The listing builds one solid part. Answer for the finished solid, in the listing's coordinates (mm). Face numbers are marked on the shaded views. A direction names the side the tool comes from. Coordinates: 2 decimals unless noted, no trailing zeros. Write each loop counter-clockwise with the first axis right and the second up, starting at its lowest first coordinate (ties: lowest second). Pieces come first, ordered by that corner, then holes. Notation, with made-up numbers: M 75.25,-32.5 L 87.25,-32.5 A10 cw 87.25,-21.5 Z; hole C 27,60.5 d3. An arc over 180 degrees is marked long. Put each result on its own line as item: value. Start each with the question number.
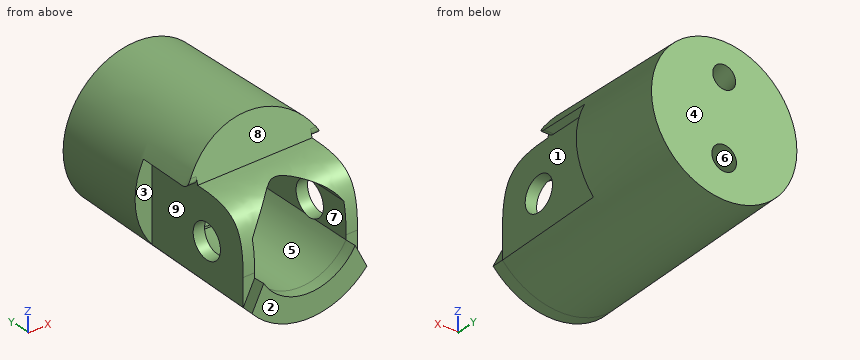
```python
from build123d import *
from build123d.topology import SkipClean

# Parameters (mm, degrees)
SKETCH1_R                     = 6.5
BOSS_EXTRUDE1_DEPTH           = 18
BOSS_EXTRUDE1_TAPER           = 1
BOSS_EXTRUDE1_OTHER_WAY_DEPTH = 10
BOSS_EXTRUDE1_OTHER_WAY_TAPER = -1
SKETCH2_W                     = 5.545055897
SKETCH2_H                     = 10
CUT_EXTRUDE1_DEPTH            = 22.497594206
CUT_EXTRUDE2_DEPTH            = 23.378552983
CUT_EXTRUDE2_DEPTH_BACK       = 23.378552983
CUT_EXTRUDE3_DEPTH            = 23.378552983
CUT_EXTRUDE3_DEPTH_BACK       = 23.378552983
SKETCH4_R                     = 1.5
FILLET1_SIZE                  = 5
CUT_EXTRUDE4_DEPTH            = 21.268192633
CUT_EXTRUDE4_DEPTH_BACK       = 21.268192633
SKETCH5_W                     = 18.469746175
SKETCH5_H                     = 12.695602453
CUT_EXTRUDE5_DEPTH            = 10
BOSS_EXTRUDE3_DEPTH           = 1
BOSS_EXTRUDE3_DRAFT           = -1
SKETCH11_R                    = 1.5
CUT_EXTRUDE7_DEPTH            = 15.423347107
CUT_EXTRUDE7_DRAFT            = -3
SKETCH12_R                    = 1.5
SKETCH13_R                    = 1


with BuildPart() as part:
    # Sketch1 → Boss-Extrude1 (new body)
    with BuildSketch(Plane(origin=(0, 0, 0), x_dir=(1, 0, 0), z_dir=(0, 1, 0))):
        Circle(SKETCH1_R)
    extrude(amount=BOSS_EXTRUDE1_DEPTH, taper=BOSS_EXTRUDE1_TAPER)

    # Sketch1 → Boss-Extrude1 other way (add)
    with BuildSketch(Plane(origin=(0, 0, 0), x_dir=(1, 0, 0), z_dir=(0, 1, 0))):
        Circle(SKETCH1_R)
    extrude(amount=-BOSS_EXTRUDE1_OTHER_WAY_DEPTH, taper=BOSS_EXTRUDE1_OTHER_WAY_TAPER)

    # Sketch2 → Cut-Extrude1 (cut, through all)
    with BuildSketch(Plane.XY.offset(3)):
        with Locations((-7.772527949, -5)):
            Rectangle(SKETCH2_W, SKETCH2_H)
        with Locations((7.772527949, -5)):
            Rectangle(SKETCH2_W, SKETCH2_H)
    extrude(amount=-CUT_EXTRUDE1_DEPTH, mode=Mode.SUBTRACT)

    # Sketch3 → Cut-Extrude2 (cut, two sides: drawn at the far end of the back side and taken through both)
    with BuildSketch(Plane(origin=(5, 0, 0), x_dir=(0, 0, -1), z_dir=(1, 0, 0)).offset(-CUT_EXTRUDE2_DEPTH_BACK)):
        Polygon((-3, -10), (-3, -5), (-18.921941618, -0.733728602), (-18.921941618, -10), align=None)
    extrude(amount=CUT_EXTRUDE2_DEPTH + CUT_EXTRUDE2_DEPTH_BACK, mode=Mode.SUBTRACT)

    # Sketch4 → Cut-Extrude3 (cut, two sides: drawn at the far end of the back side and taken through both)
    with BuildSketch(Plane(origin=(5, 0, 0), x_dir=(0, 0, -1), z_dir=(1, 0, 0)).offset(-CUT_EXTRUDE3_DEPTH_BACK)):
        with Locations(Location((1, -6, 0), (0, 0, 270))):
            Circle(SKETCH4_R)
    extrude(amount=CUT_EXTRUDE3_DEPTH + CUT_EXTRUDE3_DEPTH_BACK, mode=Mode.SUBTRACT)

    # Fillet1
    # a fillet whose section is not a circle: 5 mm, written as the material it takes off along each edge
    with BuildSketch(Plane(origin=(17.5, -10, 3), x_dir=(0, 0, -1), z_dir=(-1, 0, 0))) as fillet1_piece_1:
        with BuildLine():
            Bezier((FILLET1_SIZE, 0), (0, 0), (0, -FILLET1_SIZE), weights=[1, 1.5, 1])
            Line((0, -FILLET1_SIZE), (0, 0))
            Line((0, 0), (FILLET1_SIZE, 0))
        make_face()
    extrude(amount=35, mode=Mode.SUBTRACT)

    # Fillet2
    # a fillet whose section is not a circle: 10, 5 mm, written as the material it takes off along each edge
    with BuildSketch(Plane(origin=(0, 18, 0), x_dir=(1, 0, 0), z_dir=(0, 0, -1))) as fillet2_piece_1:
        with BuildLine():
            Bezier((6.358836316, 9.912737968), (6.185808831, 0), (1.35959784, 0), weights=[1, 0.818181818, 1])
            Line((1.35959784, 0), (6.185808831, 0))
            Line((6.185808831, 0), (6.358836316, 9.912737968))
        make_face()
    revolve(axis=Axis((0, 18, 0), (0, -1, 0)), mode=Mode.SUBTRACT)

    # Sketch5 → Cut-Extrude4 (cut, two sides: drawn at the far end of the back side and taken through both)
    with BuildSketch(Plane(origin=(0, 0, 0), x_dir=(0, 0, -1), z_dir=(1, 0, 0)).offset(-CUT_EXTRUDE4_DEPTH_BACK)):
        with Locations((0.914582981, 14.435063259)):
            Rectangle(SKETCH5_W, SKETCH5_H)
    extrude(amount=CUT_EXTRUDE4_DEPTH + CUT_EXTRUDE4_DEPTH_BACK, mode=Mode.SUBTRACT)

    # Sketch6 → Cut-Extrude5 (cut)
    with BuildSketch(Plane.XZ.offset(10)):
        with BuildLine():
            Line((-4, -2.418971635), (-4, 0.581028365))
            ThreePointArc((-4, 0.581028365), (0, 2.836607379), (4, 0.581028365))
            Line((4, 0.581028365), (4, -2.418971635))
            ThreePointArc((4, -2.418971635), (0, -4.674550649), (-4, -2.418971635))
        make_face()
    extrude(amount=-CUT_EXTRUDE5_DEPTH, mode=Mode.SUBTRACT)

    # Fillet3
    # a fillet whose section is not a circle: 0.5 mm, written as the material it takes off along each edge
    with BuildSketch(Plane(origin=(5, -5, 3), x_dir=(0, 1, 0), z_dir=(1, 0, 0))) as fillet3_piece_1:
        with BuildLine():
            Bezier((0.651612686, 0), (0, 0), (0.168649773, 0.629409523), weights=[1, 1, 1])
            Line((0.168649773, 0.629409523), (0, 0))
            Line((0, 0), (0.651612686, 0))
        make_face()
    extrude(amount=2.493517729, mode=Mode.SUBTRACT)
    with BuildSketch(Plane(origin=(-7.493517729, -5, 3), x_dir=(0, 0.258819045102518, 0.9659258262890691), z_dir=(1, 0, 0))) as fillet3_piece_2:
        with BuildLine():
            Bezier((0.651612686, 0), (0, 0), (0.168649773, -0.629409523), weights=[1, 1, 1])
            Line((0.168649773, -0.629409523), (0, 0))
            Line((0, 0), (0.651612686, 0))
        make_face()
    extrude(amount=2.493517729, mode=Mode.SUBTRACT)


with BuildPart() as boss_extrude3_tool:
    # Sketch9 → Boss-Extrude3 (with draft: the straight prism first)
    with BuildSketch(Plane.XZ.offset(10)):
        with BuildLine():
            Line((-4, -2.418971635), (-5, -4.421495943))
            ThreePointArc((-5, -4.421495943), (0, -6.674550649), (5, -4.421495943))
            Line((5, -4.421495943), (4, -2.418971635))
            ThreePointArc((4, -2.418971635), (0, -4.674550649), (-4, -2.418971635))
        make_face()
    extrude(amount=BOSS_EXTRUDE3_DEPTH)
    # Boss-Extrude3: the draft: its side faces are tilted about the plane it starts from
    boss_extrude3_sides = [boss_extrude3_tool.faces().sort_by_distance(p)[0] for p in [
        (0, -10.5, -6.674550649),
        (4.5, -10.5, -3.420233789),
        (0, -10.5, -4.674550649),
        (-4.5, -10.5, -3.420233789),
    ]]
    draft(boss_extrude3_sides, Plane.XZ.offset(10), BOSS_EXTRUDE3_DRAFT)


with BuildPart() as part_1:
    add(part.part)

    # Boss-Extrude3: add boss_extrude3_tool
    add(boss_extrude3_tool.part)


with BuildPart() as cut_extrude7_tool:
    # Sketch11 → Cut-Extrude7 (with draft: the straight prism first)
    with BuildSketch(Plane.XZ):
        with Locations((0, -3)):
            Circle(SKETCH11_R)
    extrude(amount=-CUT_EXTRUDE7_DEPTH)
    # Cut-Extrude7: the draft: its side faces are tilted about the plane it starts from
    cut_extrude7_sides = [cut_extrude7_tool.faces().sort_by_distance(p)[0] for p in [
        (-1.5, 7.711673554, -3),
    ]]
    draft(cut_extrude7_sides, Plane.XZ, CUT_EXTRUDE7_DRAFT)


with BuildPart() as part_2:
    add(part_1.part)

    # Cut-Extrude7: cut by cut_extrude7_tool
    add(cut_extrude7_tool.part, mode=Mode.SUBTRACT)

    # Sketch12 → Cut-Loft1 section 0
    with SkipClean():  # the faces are left unmerged after this step: merging them gives an invalid solid
        with BuildSketch(Plane.XZ):
            with Locations((0, 1)):
                Circle(SKETCH12_R)
        # Sketch13 → Cut-Loft1 section 1
        with BuildSketch(Plane(origin=(0, 8.087262032, 0), x_dir=(1, 0, 0), z_dir=(0, 1, 0))):
            with Locations((0, -3.5)):
                Circle(SKETCH13_R)
        loft(mode=Mode.SUBTRACT)


solid = part_2.part
```
1) A cutting plane is placed at A-A on y = -0.25. Write down the section's boundary in (x, z).
2) Determine the mould class of the marked faces 6, 7, 8 and 9 for opening direction X: +X half, -X half, draft (parallel to the pull), parting line (faces both ways), or undercut.
3) Given pin 1 Ø4 at (y, z) = (-5, -0.5) entering from -X; pin 2 Ø0.9 at (x, y) = (5.5, -1.5) entering from -Z; pin 3 Ø1.2 at (x, z) = (-5.5, 1) entering from -Y, each flat-ended and moving along its own axis, determine where each tip first touches the part or whether it passes through.
4) A cutting plane is placed at B-B on z = 0. State how many separate pieces and enclosed holes the cut face has, then the cut area to 3 significant figures.
5) For the marked faces 1, 2, 3, 4 and 5, determine the directions among +Z, -Z, +X, -X, +Y, -Y from which every point of the face is accessible in a straight line to the end or side of a thin tool.
6) Straight lines are drawn through the part: probe 1 along X at (y, z) = (-0.25, -0.5); probe 2 along Z at (x, y) = (-0.5, 2.25); probe 3 along Z at (x, y) = (3, -7.25). For each, find the intervals that lie inside material, in ascending order.
Answers follow:
1. outline: M -5.77,3 L -5,3 L -5,-4.16 A6.5 ccw 5,-4.16 L 5,3 L 5.77,3 A6.5 ccw Z; hole M -4,-2.42 A4.67 ccw 4,-2.42 L 4,0.58 A4.67 ccw -4,0.58 Z
2. face 6: undercut
2. face 7: undercut
2. face 8: draft
2. face 9: -X half
3. pin 1: stops at x = -5
3. pin 2: stops at z = 3
3. pin 3: stops at y = -9.73
4. separate pieces: 3
4. enclosed holes: 0
4. area: 117 mm²
5. face 1: -Z, +X, -Y
5. face 2: +Z, -Z, +X, -X, -Y
5. face 3: -Z, -X, -Y
5. face 4: +Z, -Z, +X, -X, +Y
5. face 5: none
6. probe 1: x = -5 to -4, 4 to 5
6. probe 2: z = -6.44 to -4.29, -1.71 to 0.43, 2.96 to 6.44
6. probe 3: z = -5.91 to -3.58, 1.75 to 2.83
